Here's how the part is built. I have some questions about the finished solid (model axes, mm). Give positions to 0.01 mm unless a question says otherwise; leave off trailing zeros. Loops run counter-clockwise (first coordinate to the right, second up) from the corner with the lowest first, then second, coordinate; pieces in that order, holes last. Notation, with made-up numbers: (14.25, 23) - (58.25, 23) arc R12 cw to (58.25, 42) - close; hole circle Ø8 at (-18.5, -24). An arc over 180 degrees is marked (long way). Use one line per item in the form item = value.
from build123d import *

# Parameters (mm, degrees)
SKETCH1_W           = 153
SKETCH1_H           = 420
BOSS_EXTRUDE1_DEPTH = 2
CUT_EXTRUDE1_REACH  = 225.509
SKETCH2_W           = 43
SKETCH2_H           = 398
CUT_EXTRUDE2_REACH  = 225.509
SKETCH3_R           = 3


with BuildPart() as part:
    # Sketch1 → Boss-Extrude1 (new body)
    with BuildSketch(Plane.XY):
        Rectangle(SKETCH1_W, SKETCH1_H)
    extrude(amount=BOSS_EXTRUDE1_DEPTH)

    # Sketch2 → Cut-Extrude1 (cut, up to next)
    with BuildSketch(Plane(origin=(0, 0, 0), x_dir=(-1, 0, 0), z_dir=(0, 0, -1)), mode=Mode.PRIVATE) as cut_extrude1_sk1:
        with Locations((-25, 11)):
            Rectangle(SKETCH2_W, SKETCH2_H)
    cut_extrude1_tool1 = extrude(cut_extrude1_sk1.sketch, amount=-CUT_EXTRUDE1_REACH, mode=Mode.PRIVATE) & part.part
    add(cut_extrude1_tool1.solids().sort_by_distance((25, 11, 0))[0], mode=Mode.SUBTRACT)

    # Sketch3 → Cut-Extrude2 (cut, up to next)
    with BuildSketch(Plane(origin=(0, 0, 0), x_dir=(-1, 0, 0), z_dir=(0, 0, -1)), mode=Mode.PRIVATE) as cut_extrude2_sk1:
        with Locations((-62, 202)):
            Circle(SKETCH3_R)
    cut_extrude2_tool1 = extrude(cut_extrude2_sk1.sketch, amount=-CUT_EXTRUDE2_REACH, mode=Mode.PRIVATE) & part.part
    # Sketch3 → Cut-Extrude2 (cut, up to next)
    with BuildSketch(Plane(origin=(0, 0, 0), x_dir=(-1, 0, 0), z_dir=(0, 0, -1)), mode=Mode.PRIVATE) as cut_extrude2_sk2:
        with Locations((-62, -199)):
            Circle(SKETCH3_R)
    cut_extrude2_tool2 = extrude(cut_extrude2_sk2.sketch, amount=-CUT_EXTRUDE2_REACH, mode=Mode.PRIVATE) & part.part
    # Sketch3 → Cut-Extrude2 (cut, up to next)
    with BuildSketch(Plane(origin=(0, 0, 0), x_dir=(-1, 0, 0), z_dir=(0, 0, -1)), mode=Mode.PRIVATE) as cut_extrude2_sk3:
        with Locations((62, 202)):
            Circle(SKETCH3_R)
    cut_extrude2_tool3 = extrude(cut_extrude2_sk3.sketch, amount=-CUT_EXTRUDE2_REACH, mode=Mode.PRIVATE) & part.part
    # Sketch3 → Cut-Extrude2 (cut, up to next)
    with BuildSketch(Plane(origin=(0, 0, 0), x_dir=(-1, 0, 0), z_dir=(0, 0, -1)), mode=Mode.PRIVATE) as cut_extrude2_sk4:
        with Locations((62, -199)):
            Circle(SKETCH3_R)
    cut_extrude2_tool4 = extrude(cut_extrude2_sk4.sketch, amount=-CUT_EXTRUDE2_REACH, mode=Mode.PRIVATE) & part.part
    add(cut_extrude2_tool1.solids().sort_by_distance((62, 202, 0))[0], mode=Mode.SUBTRACT)
    add(cut_extrude2_tool2.solids().sort_by_distance((62, -199, 0))[0], mode=Mode.SUBTRACT)
    add(cut_extrude2_tool3.solids().sort_by_distance((-62, 202, 0))[0], mode=Mode.SUBTRACT)
    add(cut_extrude2_tool4.solids().sort_by_distance((-62, -199, 0))[0], mode=Mode.SUBTRACT)


solid = part.part
(1) If I drill on probe 1 along Y at (x, z) = (-62, 1.1); probe 2 along X at (y, z) = (-199, 1.45); probe 3 along X at (y, z) = (-41.5, 1.85), over which ranges is the centre line in solid material (lowest first)?
Geometry says:
probe_1 = -210 to -202, -196 to 199, 205 to 210
probe_2 = -76.5 to -65, -59 to 59, 65 to 76.5
probe_3 = -76.5 to 3.5, 46.5 to 76.5
(2) If we section it at B-B (z = 0.45): List the corners of the cut face in (x, y) for me, plus the area to 3 significant figures.
Geometry says:
outline = (-76.5, -210) - (76.5, -210) - (76.5, 210) - (46.5, 210) - (46.5, -188) - (3.5, -188) - (3.5, 210) - (-76.5, 210) - close; hole circle Ø6 at (-62, -199); hole circle Ø6 at (-62, 202); hole circle Ø6 at (62, -199); hole circle Ø6 at (62, 202)
area = 47,000 mm²
(3) If we section it at C-C (x = 37.5): List the corners of the cut face in (y, z) for me, plus the area to 3 significant figures.
Geometry says:
outline = (-210, 0) - (-188, 0) - (-188, 2) - (-210, 2) - close
area = 44.0 mm²
(4) For P1, Ø3.5, axis at x = -62, y = 202, coming from the +Z side, with a flat end and sliding along its axis, tell me the tip position at first contact or that it passes through.
Geometry says:
P1 = through
(5) If we section it at A-A (y = -81.5): List the corners of the cut face in (x, z) for me.
Geometry says:
outline = (-76.5, 0) - (3.5, 0) - (3.5, 2) - (-76.5, 2) - close; (46.5, 0) - (76.5, 0) - (76.5, 2) - (46.5, 2) - close
